from build123d import *

# Parameters (mm, degrees)
F0_R     = 1.55
F0_R_2   = 1.625
F1_DEPTH = 3
F2_W     = 28.2
F2_H     = 28.2
F3_DEPTH = 3
F5_DEPTH = 25
F7_DEPTH = 25
F8_R     = 1


with BuildPart() as f1:
    # F0 (on Top) → F1 (new body)
    with BuildSketch(Plane.XY):
        with BuildLine():
            Line((58, 24), (58, 41.313006))
            ThreePointArc((58, 41.313006), (70.547763, 63.673914), (44.920157, 64.5))
            Line((44.920157, 64.5), (0, 64.5))
            Line((0, 64.5), (-44.920157, 64.5))
            ThreePointArc((-44.920157, 64.5), (-70.547763, 63.673914), (-58, 41.313006))
            Line((-58, 41.313006), (-58, 0))
            Line((-58, 0), (-58, -41.313006))
            ThreePointArc((-58, -41.313006), (-70.547763, -63.673914), (-44.920157, -64.5))
            Line((-44.920157, -64.5), (0, -64.5))
            Line((0, -64.5), (44.920157, -64.5))
            ThreePointArc((44.920157, -64.5), (70.547763, -63.673914), (58, -41.313006))
            Line((58, -41.313006), (58, -24))
            Line((58, -24), (99, -24))
            Line((99, -24), (99, 24))
            Line((99, 24), (58, 24))
        make_face()
        with Locations((-58.427906, -56.837072)):
            Circle(F0_R, mode=Mode.SUBTRACT)
        with Locations((-42, -59.5)):
            Circle(F0_R_2, mode=Mode.SUBTRACT)
        with Locations((-53, -40)):
            Circle(F0_R_2, mode=Mode.SUBTRACT)
        with Locations((42, -59.5)):
            Circle(F0_R_2, mode=Mode.SUBTRACT)
        with Locations((53, -40)):
            Circle(F0_R_2, mode=Mode.SUBTRACT)
        with Locations((58.427906, -56.837072)):
            Circle(F0_R, mode=Mode.SUBTRACT)
        with Locations((53, -19)):
            Circle(F0_R_2, mode=Mode.SUBTRACT)
        with Locations((91, -19)):
            Circle(F0_R_2, mode=Mode.SUBTRACT)
        Polygon((39.079843, 54.5), (48, 38.686994), (48, 0), (48, -38.686994), (39.079843, -54.5), (0, -54.5), (-39.079843, -54.5), (-48, -38.686994), (-48, 0), (-48, 38.686994), (-39.079843, 54.5), (0, 54.5), align=None, mode=Mode.SUBTRACT)
        with Locations((-53, 40)):
            Circle(F0_R_2, mode=Mode.SUBTRACT)
        with Locations((-58.427906, 56.837072)):
            Circle(F0_R, mode=Mode.SUBTRACT)
        with Locations((-42, 59.5)):
            Circle(F0_R_2, mode=Mode.SUBTRACT)
        with Locations((53, 19)):
            Circle(F0_R_2, mode=Mode.SUBTRACT)
        Polygon((86, 14), (86, -14), (58, -14), (58, 0), (58, 14), align=None, mode=Mode.SUBTRACT)
        with Locations((91, 19)):
            Circle(F0_R_2, mode=Mode.SUBTRACT)
        with Locations((53, 40)):
            Circle(F0_R_2, mode=Mode.SUBTRACT)
        with Locations((42, 59.5)):
            Circle(F0_R_2, mode=Mode.SUBTRACT)
        with Locations((58.427906, 56.837072)):
            Circle(F0_R, mode=Mode.SUBTRACT)
    extrude(amount=F1_DEPTH)

    # F2 (on Top) → F3 (join)
    with BuildSketch(Plane.XY):
        with Locations((72, 0)):
            Rectangle(F2_W, F2_H)
    extrude(amount=F3_DEPTH)

    # F4 (on face) → F5 (cut)
    with BuildSketch(Plane.XY.offset(3)):
        with BuildLine():
            Line((99, -10), (98, -10))
            ThreePointArc((98, -10), (97, -11), (98, -12))
            Line((98, -12), (99, -12))
            Line((99, -12), (99, -10))
        make_face()
    extrude(amount=-F5_DEPTH, mode=Mode.SUBTRACT)

    # F6 (on Top) → F7 (cut)
    with BuildSketch(Plane.XY):
        with BuildLine():
            Line((1.5, 54.5), (1.5, 56))
            ThreePointArc((1.5, 56), (0, 57.5), (-1.5, 56))
            Line((-1.5, 56), (-1.5, 54.5))
            Line((-1.5, 54.5), (1.5, 54.5))
        make_face()
    extrude(amount=F7_DEPTH, mode=Mode.SUBTRACT)

    # F8
    f8_edges = [f1.edges().sort_by_distance(p)[0] for p in [
        (-1.5, 54.5, 1.5),
        (1.5, 54.5, 1.5),
    ]]
    fillet(f8_edges, radius=F8_R)


solid = f1.part
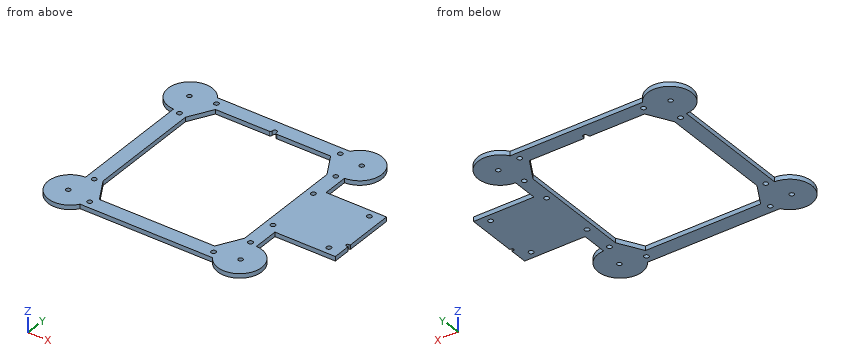
Here's how the part is built. I have some questions about the finished solid (model axes, mm). Coordinates: 2 decimals unless noted, no trailing zeros. Order: outer loops, then holes, each group sorted by start corner. A loop starts at its lowest first (then second) coordinate and runs counter-clockwise, first axis right, second up.
Item 1: For P1, Ø1.5, axis at y = 38, z = 1, coming from the -X side; P2, Ø4, axis at x = 53, y = -19, coming from the +Z side; P3, Ø1.9, axis at x = -53, y = 40, coming from the -Z side; P4, Ø0.8, axis at x = 98.5, z = 1, coming from the -Y side, each with a flat end and sliding along its axis, tell me the tip position at first contact or that it passes through.
Result sheet:
P1: stops at x = -58
P2: stops at z = 3
P3: passes through
P4: stops at y = -24
Item 2: I need wall thicknesses on line 1 (Y direction, x = 91, z = 1.8) (3 decimals); line 2 (X direction, y = -29, z = 2.55); line 3 (X direction, y = -14, z = 0.5). Which ranges of each line are inside material? Lowest first, please.
Result sheet:
line 1: y = -24 to -20.625, -17.375 to 17.375, 20.625 to 24
line 2: x = -58 to -48, 48 to 58
line 3: x = -58 to -48, 48 to 99
Item 3: If we section it at B-B on x = 82.5: List the corners of the cut face in (y, z) for me, plus the area to 3 significant figures.
Result sheet:
outline: (-24, 0) - (24, 0) - (24, 3) - (-24, 3) - close
area: 144 mm2
Item 4: If we section it at C-C on z = 2.1: State how many separate pieces and enclosed holes the cut face has, plus the area to 3 significant figures.
Result sheet:
separate pieces: 1
enclosed holes: 17
area: 8,210 mm2
Item 5: If we section it at A-A on x = 27.5: List the corners of the cut face in (y, z) for me, plus the area to 3 significant figures.
Result sheet:
outline: (-64.5, 0) - (-54.5, 0) - (-54.5, 3) - (-64.5, 3) - close; (54.5, 0) - (64.5, 0) - (64.5, 3) - (54.5, 3) - close
area: 60.0 mm2
